Work out the finished part from the listing and answer in its coordinate system (mm). Coordinates: 2 decimals unless noted, no trailing zeros. Write each loop counter-clockwise with the first axis right and the second up, starting at its lowest first coordinate (ties: lowest second). Pieces come first, ordered by that corner, then holes. Notation, with made-up numbers: M 61,87.25 L 116,87.25 A23 cw 116,110.25 Z; hole C 22,31.5 d3. An arc over 180 degrees is marked long. Answer as CSV lines item,"result". Start each with the question number.
(1) Find the intervals of material crossed by L1, parallel to Y at x = -2, z = 207.5; L2, parallel to Y at x = 12.5, z = 52, in increasing order. Write a range as [from, to].
(2) A cutting plane is placed at B-B on x = 0.5. Give the vertices of the cut face in (y, z), then the cut area to 3 significant figures.
(3) A flat-ended cylindrical pin translates along its axis: P1, Ø6, axis at x = 12.5, y = -9.5, coming from the +Z side. Find the tip coordinate at first contact, or state that the pin passes through.
(4) A cutting plane is placed at A-A on y = -5. Give the vertices of the cut face in (x, z).
(5) A cutting plane is placed at C-C on z = 746. Give the vertices of the cut face in (x, y), then the cut area to 3 significant figures.
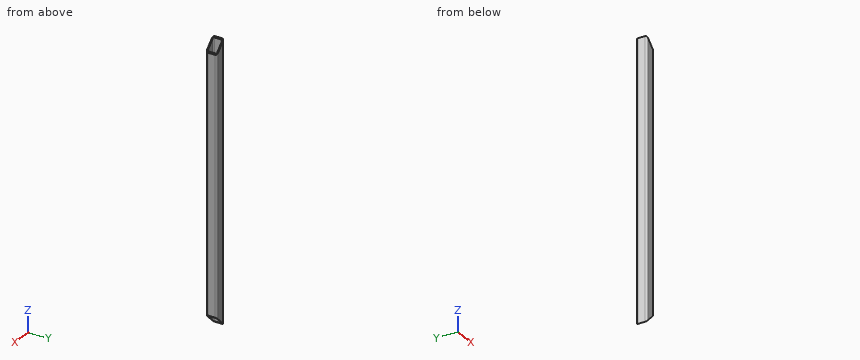
Autodesk Inventor part; units mm, degrees
ref_plane "Počáteční rovina" through (0, 0, 0) normal (0, 0, 1) x (1, 0, 0)
ref_plane "Koncová rovina" through (0, 0, 875) normal (0, 0, 1) x (1, 0, 0)
ref_plane "YZ Plane" through (0, 0, 0) normal (1, 0, 0) x (0, 1, 0)
ref_plane "Počáteční rovina" through (0, 0, 0) normal (0, 0, 1) x (1, 0, 0)
ref_plane "Koncová rovina" through (0, 0, 875) normal (0, 0, 1) x (1, 0, 0)
sketch "Náčrt1" plane through (0, 0, 0) normal (0, 0, 1) x (1, 0, 0)
  line L0 (-11.5, 17.5) -> (11.5, 17.5)
  line L1 (17.5, 11.5) -> (17.5, -11.5)
  line L2 (11.5, -17.5) -> (-11.5, -17.5)
  line L3 (-17.5, -11.5) -> (-17.5, 11.5)
  arc A0 (-11.5, 17.5) -> (-17.5, 11.5) centre (-11.5, 11.5) ccw
  arc A1 (17.5, 11.5) -> (11.5, 17.5) centre (11.5, 11.5) ccw
  arc A2 (11.5, -17.5) -> (17.5, -11.5) centre (11.5, -11.5) ccw
  arc A3 (-17.5, -11.5) -> (-11.5, -17.5) centre (-11.5, -11.5) ccw
  line L4 (-21.8698, 0) -> (21.8698, 0) construction
  line L5 (0, -21.8698) -> (0, 21.8698) construction
  arc A4 (-11.5, 14.5) -> (-14.5, 11.5) centre (-11.5, 11.5) ccw
  line L6 (-11.5, 14.5) -> (11.5, 14.5)
  arc A5 (14.5, 11.5) -> (11.5, 14.5) centre (11.5, 11.5) ccw
  line L7 (14.5, 11.5) -> (14.5, -11.5)
  arc A6 (11.5, -14.5) -> (14.5, -11.5) centre (11.5, -11.5) ccw
  line L8 (11.5, -14.5) -> (-11.5, -14.5)
  arc A7 (-14.5, -11.5) -> (-11.5, -14.5) centre (-11.5, -11.5) ccw
  line L9 (-14.5, -11.5) -> (-14.5, 11.5)
  point P0 (-17.5, 17.5)
  point P1 (17.5, -17.5)
  point P2 (17.5, 17.5)
  dimension "b" = 35
  dimension "msp_r" = 6
  dimension "d8" = 17.5
  dimension "d9" = 17.5
  dimension "d10" = 3
extrude "Těleso" add sketch "Náčrt1" along normal up to surface (875 mm away) from surface at 0
sketch "Sketch2" plane through (0, 0, 0) normal (0, 0, 1) x (1, 0, 0)
  line L0 (0, 0) -> (10, 0)
ref_plane "Work Plane3" through (0, 0, 0) normal (0, -1, 0) x (1, 0, 0)
sketch "Sketch3" plane through (0, 0, 0) normal (0, -1, 0) x (1, 0, 0)
  line L0 (-2, 0) -> (12, 0)
  line L1 (-2, 875) -> (12, 875)
  dimension "d14" = 875
sketch "Náčrt4" plane through (11.5, 17.5, 875) normal (0, 1, 0) x (1, 0, 0)
  line L0 (-29, 875) -> (-29, 0) construction
  line L1 (6, 875) -> (6, 0) construction
  line L2 (-29, 875) -> (6, 875)
  line L3 (6, 875) -> (6, 840)
  line L4 (-29, 875) -> (-29, 0) construction
  line L5 (6, 840) -> (-29, 875)
  line L6 (-29, 0) -> (6, 35)
  line L7 (6, 875) -> (6, 0) construction
  line L8 (6, 35) -> (6, 0)
  line L9 (6, 0) -> (-29, 0)
  point P0 (-11.5, 875)
  dimension "d15" = 45
  dimension "d16" = 45
extrude "Vysunutí2" cut sketch "Náčrt4" against normal through all
equation "\"msp_r\" = 2 * ParT"
equation "\"d8\" = d9"
equation "\"d9\" = 0.5 * b"
equation "\"d10\" = ParT"
equation "\"G_OFFSET_START\" = 0"
equation "\"G_OFFSET_END\" = 0"
equation "\"d12\" = G_OFFSET_END + B_L"
equation "\"G_L\" = d14"
equation "\"B_L\" = 875"
properties part number "CSN 426935 - 35x35x3-875" material "Nerezová ocel"
Here are the results:
1,L1,"y = [-17.5, -14.5], [14.5, 17.5]"
1,L2,"y = [-17.42, -14.33], [14.33, 17.42]"
2,outline,"M -17.5,18 L -14.5,18 L -14.5,857 L -17.5,857 Z; M 14.5,18 L 17.5,18 L 17.5,857 L 14.5,857 Z"
2,area,"5,030 mm^2"
3,P1,"stops at z = 843.01"
4,outline,"M -17.5,0 L -14.5,3 L -14.5,872 L -17.5,875 Z; M 14.5,32 L 17.5,35 L 17.5,840 L 14.5,843 Z"
5,outline,"M -17.5,-11.5 A6 ccw -11.5,-17.5 L 11.5,-17.5 A6 ccw 17.5,-11.5 L 17.5,11.5 A6 ccw 11.5,17.5 L -11.5,17.5 A6 ccw -17.5,11.5 Z; hole M -14.5,-11.5 A3 ccw -11.5,-14.5 L 11.5,-14.5 A3 ccw 14.5,-11.5 L 14.5,11.5 A3 ccw 11.5,14.5 L -11.5,14.5 A3 ccw -14.5,11.5 Z"
5,area,"361 mm^2"
